Input: part model. Units: mm. Frame: model coordinates. Face numbers are marked on the shaded views. A direction names the side the tool comes from. Coordinates: 2 decimals unless noted, no trailing zeros. Order: outer loops, then holes, each group sorted by start corner. A loop starts at its lowest first (then second) coordinate and runs counter-clockwise, first axis right, second up. Notation, with made-up numbers: (-0.75, 33.25) -> (4.25, 33.25) arc R16 cw to (4.25, 49.25) -> close; hole circle Ø10 at (56.25, -15.75). An arc over 180 degrees is marked (long way). Use CSV: the item, a comma, the result in double quotes. Start each with the question number.
```python
from build123d import *

# Parameters (mm, degrees)
SKETCH1_W           = 495
SKETCH1_H           = 150
BOSS_EXTRUDE1_DEPTH = 30
SKETCH2_R           = 17.5
SKETCH2_W           = 55
SKETCH2_H           = 55
CUT_EXTRUDE1_DEPTH  = 20
CUT_EXTRUDE2_DEPTH  = 25
CUT_EXTRUDE2_TAPER  = 30
SKETCH5_W           = 55
SKETCH5_H           = 55
SKETCH5_W_2         = 35
SKETCH5_H_2         = 35
CUT_EXTRUDE3_DEPTH  = 20
FILLET1_R           = 20
SKETCH8_W           = 59
SKETCH8_H           = 59
SKETCH8_W_2         = 55
SKETCH8_H_2         = 55
BOSS_EXTRUDE2_DEPTH = 2
SKETCH9_R           = 19.5
SKETCH9_R_2         = 17.5
BOSS_EXTRUDE3_DEPTH = 2
BOSS_EXTRUDE4_DEPTH = 2
SKETCH11_W          = 59
SKETCH11_H          = 59
SKETCH11_W_2        = 55
SKETCH11_H_2        = 55
BOSS_EXTRUDE6_DEPTH = 2
SKETCH12_W          = 39
SKETCH12_H          = 39
SKETCH12_W_2        = 35
SKETCH12_H_2        = 35
BOSS_EXTRUDE7_DEPTH = 2
SKETCH13_R          = 19.5
SKETCH13_R_2        = 17.5
BOSS_EXTRUDE8_DEPTH = 2


with BuildPart() as part:
    # Sketch1 → Boss-Extrude1 (new body)
    with BuildSketch(Plane(origin=(0, 0, 0), x_dir=(1, 0, 0), z_dir=(0, 1, 0))):
        Rectangle(SKETCH1_W, SKETCH1_H)
    extrude(amount=BOSS_EXTRUDE1_DEPTH)

    # Sketch2 → Cut-Extrude1 (cut)
    with BuildSketch(Plane(origin=(0, 30, 0), x_dir=(1, 0, 0), z_dir=(0, 1, 0))):
        with Locations((-115, 0)):
            Circle(SKETCH2_R)
        with Locations((-190, 0)):
            Rectangle(SKETCH2_W, SKETCH2_H)
    extrude(amount=-CUT_EXTRUDE1_DEPTH, mode=Mode.SUBTRACT)

    # Sketch4 → Cut-Extrude2 (cut)
    with BuildSketch(Plane(origin=(0, 30, 0), x_dir=(1, 0, 0), z_dir=(0, 1, 0))):
        Polygon((-67.5, 14.287926899), (-67.5, -14.712073101), (-46.782926899, -35.005), (-17.782926899, -35.005), (2.51, -14.287926899), (2.51, 14.712073101), (-18.207073101, 35.005), (-47.207073101, 35.005), align=None)
    extrude(amount=-CUT_EXTRUDE2_DEPTH, taper=CUT_EXTRUDE2_TAPER, mode=Mode.SUBTRACT)

    # Sketch5 → Cut-Extrude3 (cut)
    with BuildSketch(Plane(origin=(0, 30, 0), x_dir=(1, 0, 0), z_dir=(0, 1, 0))):
        with Locations((60.01, 0)):
            Rectangle(SKETCH5_W, SKETCH5_H)
        with Locations((135.01, 0)):
            Rectangle(SKETCH5_W_2, SKETCH5_H_2)
    extrude(amount=-CUT_EXTRUDE3_DEPTH, mode=Mode.SUBTRACT)

    # Sketch6 → Cut-Revolve1 (revolve, cut)
    with BuildSketch(Plane(origin=(0, 30, 0), x_dir=(1, 0, 0), z_dir=(0, 1, 0))):
        with BuildLine():
            Line((217.51, 0), (182.51, 0))
            ThreePointArc((182.51, 0), (200.01, 17.5), (217.51, 0))
        make_face()
    revolve(axis=Axis((217.51, 30, 0), (-1, 0, 0)), mode=Mode.SUBTRACT)

    # Fillet1
    fillet1_edges = [part.edges().sort_by_distance(p)[0] for p in [
        (247.5, 15, 75),
        (-247.5, 15, 75),
        (-247.5, 15, -75),
        (247.5, 15, -75),
    ]]
    fillet(fillet1_edges, radius=FILLET1_R)

    # Sketch8 → Boss-Extrude2 (add)
    with BuildSketch(Plane(origin=(0, 30, 0), x_dir=(1, 0, 0), z_dir=(0, 1, 0))):
        with Locations((-190, 0)):
            Rectangle(SKETCH8_W, SKETCH8_H)
        with Locations((-190, 0)):
            Rectangle(SKETCH8_W_2, SKETCH8_H_2, mode=Mode.SUBTRACT)
    extrude(amount=BOSS_EXTRUDE2_DEPTH)

    # Sketch9 → Boss-Extrude3 (add)
    with BuildSketch(Plane(origin=(0, 30, 0), x_dir=(1, 0, 0), z_dir=(0, 1, 0))):
        with Locations((-115, 0)):
            Circle(SKETCH9_R)
        with Locations((-115, 0)):
            Circle(SKETCH9_R_2, mode=Mode.SUBTRACT)
    extrude(amount=BOSS_EXTRUDE3_DEPTH)

    # Sketch10 → Boss-Extrude4 (add)
    with BuildSketch(Plane(origin=(0, 30, 0), x_dir=(1, 0, 0), z_dir=(0, 1, 0))):
        Polygon((-48.207073101, 37.005), (-17.207073101, 37.005), (4.713237116, 15.084689783), (4.713237116, -15.915310217), (-17.207073101, -37.835620434), (-48.207073101, -37.835620434), (-70.127383317, -15.915310217), (-70.127383317, 15.084689783), align=None)
        Polygon((-47.207073101, 35.005), (-18.207073101, 35.005), (2.51, 14.712073101), (2.51, -14.287926899), (-17.782926899, -35.005), (-46.782926899, -35.005), (-67.5, -14.712073101), (-67.5, 14.287926899), align=None, mode=Mode.SUBTRACT)
    extrude(amount=BOSS_EXTRUDE4_DEPTH)

    # Sketch11 → Boss-Extrude6 (add)
    with BuildSketch(Plane(origin=(0, 30, 0), x_dir=(1, 0, 0), z_dir=(0, 1, 0))):
        with Locations((60.01, 0)):
            Rectangle(SKETCH11_W, SKETCH11_H)
        with Locations((60.01, 0)):
            Rectangle(SKETCH11_W_2, SKETCH11_H_2, mode=Mode.SUBTRACT)
    extrude(amount=BOSS_EXTRUDE6_DEPTH)

    # Sketch12 → Boss-Extrude7 (add)
    with BuildSketch(Plane(origin=(0, 30, 0), x_dir=(1, 0, 0), z_dir=(0, 1, 0))):
        with Locations((135.01, 0)):
            Rectangle(SKETCH12_W, SKETCH12_H)
        with Locations((135.01, 0)):
            Rectangle(SKETCH12_W_2, SKETCH12_H_2, mode=Mode.SUBTRACT)
    extrude(amount=BOSS_EXTRUDE7_DEPTH)

    # Sketch13 → Boss-Extrude8 (add)
    with BuildSketch(Plane(origin=(0, 30, 0), x_dir=(1, 0, 0), z_dir=(0, 1, 0))):
        with Locations((200.01, 0)):
            Circle(SKETCH13_R)
        with Locations((200.01, 0)):
            Circle(SKETCH13_R_2, mode=Mode.SUBTRACT)
    extrude(amount=BOSS_EXTRUDE8_DEPTH)


solid = part.part
```
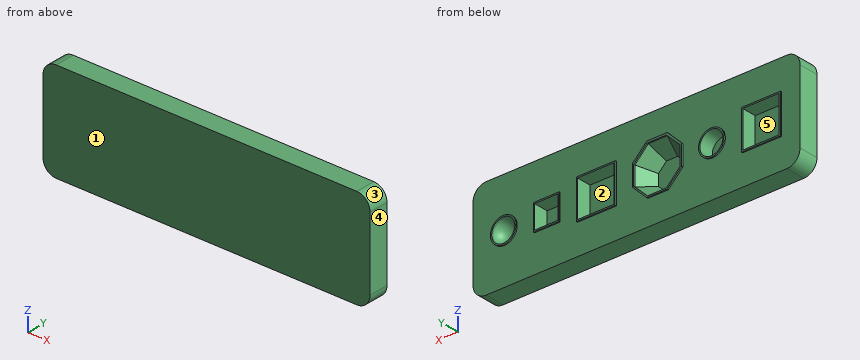
1. Section B-B on z = 43.5. Return loops of the section in (x, y), then the cut area to 4 significant figures.
2. Pull-direction query (X, two-part tool) for the marked faces 1, 2 and 3; classes: released by +X, released by -X, zero draft, split by the parting line, or undercut.
3. Section A-A on x = 200.01. Return loops of the section in (y, z), then the cut area to 3 significant figures.
4. Section C-C on x = -115. Return loops of the section in (y, z).
5. Contact query for flat-ended pins moving along their axis: P1, Ø16.5, axis at x = -178.5, z = 7.5, coming from the +Y side; P2, Ø1.6, axis at x = 132, y = 31.5, coming from the -Z side; P3, Ø1, axis at x = 53, y = 31.5, coming from the +Z side; P4, Ø1.5, axis at x = 23.5, z = -56, coming from the -Y side. Output: stop coordinate, or through.
6. Material intervals for line 1 along Z through (x, y) = (-116, 28.5); line 2 along Z through (x, y) = (33, 16.5); line 3 along Y through (x, z) = (-59.5, 30), sorted ascending.
7. Access query for the marked faces 4 and 5. Directions: +Z, -Z, +X, -X, +Y, -Y. A direction counts if a zero-diameter tool reaches every point of the face in a straight line with its end or side. Return the directions, or none.
Values follow:
1,outline,"(-247.5, 0) -> (247.5, 0) -> (247.5, 30) -> (-247.5, 30) -> close"
1,area,"14,850 mm2"
2,face 1,"zero draft"
2,face 2,"undercut"
2,face 3,"released by +X"
3,outline,"(0, -75) -> (30, -75) -> (30, -19.5) -> (32, -19.5) -> (32, -17.5) -> (30, -17.5) arc R17.5 cw to (30, 17.5) -> (32, 17.5) -> (32, 19.5) -> (30, 19.5) -> (30, 75) -> (0, 75) -> close"
3,area,"4,030 mm2"
4,outline,"(0, -75) -> (30, -75) -> (30, -19.5) -> (32, -19.5) -> (32, -17.5) -> (10, -17.5) -> (10, 17.5) -> (32, 17.5) -> (32, 19.5) -> (30, 19.5) -> (30, 75) -> (0, 75) -> close"
5,P1,"stops at y = 10"
5,P2,"stops at z = -19.5"
5,P3,"stops at z = 29.5"
5,P4,"stops at y = 0"
6,line 1,"z = -75 to -17.47, 17.47 to 75"
6,line 2,"z = -75 to -27.5, 27.5 to 75"
6,line 3,"y = 0 to 30"
7,face 4,"+Z, -Z, +X, +Y, -Y"
7,face 5,"+Y"
